from build123d import *

# Parameters (mm, degrees)
SKETCH2_R           = 7
BOSS_EXTRUDE2_DEPTH = 34
SKETCH3_R           = 5
BOSS_EXTRUDE3_DEPTH = 20
SKETCH4_R           = 3
CUT_EXTRUDE1_DEPTH  = 29


with BuildPart() as part:
    # Sketch2 → Boss-Extrude2 (new body)
    with BuildSketch(Plane(origin=(0, 0, 0), x_dir=(-1, 0, 0), z_dir=(0, 0, -1))):
        with Locations((-15.057769352, -8.761383704)):
            Circle(SKETCH2_R)
    extrude(amount=BOSS_EXTRUDE2_DEPTH)

    # Sketch3 → Boss-Extrude3 (add)
    with BuildSketch(Plane(origin=(0, 0, -34), x_dir=(-1, 0, 0), z_dir=(0, 0, -1))):
        with Locations((-15.057769352, -8.761383704)):
            Circle(SKETCH3_R)
    extrude(amount=BOSS_EXTRUDE3_DEPTH)

    # Sketch4 → Cut-Extrude1 (cut)
    with BuildSketch(Plane(origin=(0, 0, -54), x_dir=(-1, 0, 0), z_dir=(0, 0, -1))):
        with Locations(Location((-15.057769352, -8.761383704, 0), (0, 0, 180))):
            Circle(SKETCH4_R)
    extrude(amount=-CUT_EXTRUDE1_DEPTH, mode=Mode.SUBTRACT)


solid = part.part
Source: CAD feature listing. Evaluate the final solid. Frame: model axes, mm. A direction names the side the tool comes from. Round coordinates to 2 decimals unless told otherwise and drop trailing zeros. Loops run counter-clockwise (first coordinate to the right, second up) from the corner with the lowest first, then second, coordinate; pieces in that order, holes last.
Q1. Section D-D, the plane y = -10.75. Return loops of the section in (x, z), plus the area to 3 significant figures.
Q2. Access query for faces 1 (the face through (15, -9, 0)), 2 (the face through (12.37, -4.545, -43.86)). Directions: +Z, -Z, +X, -X, +Y, -Y. A direction counts if a zero-diameter tool reaches every point of the face in a straight line with its end or side. Return the directions, or none.
Q3. Section B-B, the plane x = 17.25. Return loops of the section in (y, z), plus the area to 3 significant figures.
Q4. Section A-A, the plane y = -13. Return loops of the section in (x, z), plus the area to 3 significant figures.
Q5. Section C-C, the plane z = -50. Return loops of the section in (x, y), plus the area to 3 significant figures.
Q6. Ray query, line 1 (Z direction, x = 13.75, y = -7); line 2 (Y direction, x = 16, z = -51); line 3 (Z direction, x = 14.5, y = -15). Return the intervals inside material, ascending.
Q7. First-contact query: P1, Ø6, axis at x = 14, z = -39.5, coming from the -Y side; P2, Ø3.5, axis at x = 15.06, y = -8.76, coming from the -Z side. Flat tips, straight axial feed; report the tip coordinate or a pass-through.
Solutions:
1. outline: (8.35, -34) - (10.47, -34) - (10.47, -54) - (12.81, -54) - (12.81, -25) - (17.3, -25) - (17.3, -54) - (19.65, -54) - (19.65, -34) - (21.77, -34) - (21.77, 0) - (8.35, 0) - close
1. area: 510 mm2
2. face 1: +Z, +X, -X, +Y, -Y
2. face 2: -Z
3. outline: (-15.41, -34) - (-13.26, -34) - (-13.26, -54) - (-10.81, -54) - (-10.81, -25) - (-6.71, -25) - (-6.71, -54) - (-4.27, -54) - (-4.27, -34) - (-2.11, -34) - (-2.11, 0) - (-15.41, 0) - close
3. area: 513 mm2
4. outline: (9.49, -34) - (12.41, -34) - (12.41, -54) - (17.71, -54) - (17.71, -34) - (20.63, -34) - (20.63, 0) - (9.49, 0) - close
4. area: 485 mm2
5. outline: circle Ø10 at (15.06, -8.76); hole circle Ø6 at (15.06, -8.76)
5. area: 50.3 mm2
6. line 1: z = -25 to 0
6. line 2: y = -13.67 to -11.61, -5.91 to -3.85
6. line 3: z = -34 to 0
7. P1: stops at y = -13.76
7. P2: stops at z = -25
